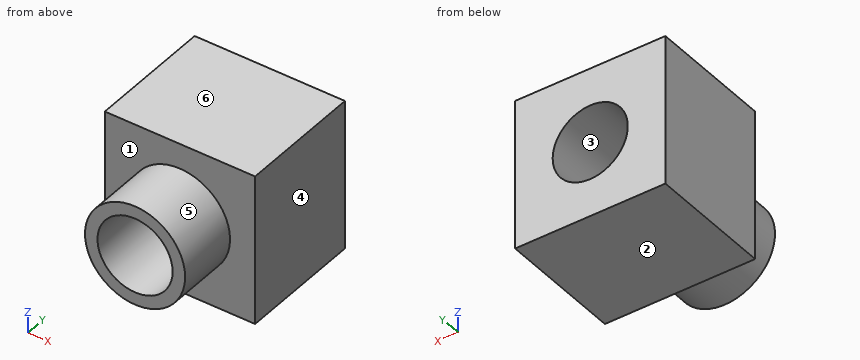
```python
from build123d import *

# Parameters (mm, degrees)
F0_W     = 600
F0_H     = 600
F1_DEPTH = 250
F2_R     = 200
F2_R_2   = 150
F3_DEPTH = 250
F4_R     = 150
F5_DEPTH = 1016


with BuildPart() as f1:
    # F0 (on Front) → F1 (new body, symmetric)
    with BuildSketch(Plane.XZ):
        Rectangle(F0_W, F0_H)
    extrude(amount=F1_DEPTH, both=True)

    # F2 (on face) → F3 (join)
    with BuildSketch(Plane.XZ.offset(250)):
        Circle(F2_R)
        Circle(F2_R_2, mode=Mode.SUBTRACT)
    extrude(amount=F3_DEPTH)

    # F4 (on face) → F5 (cut)
    with BuildSketch(Plane.XZ.offset(500)):
        Circle(F4_R)
    extrude(amount=-F5_DEPTH, mode=Mode.SUBTRACT)


solid = f1.part
```
Geometry check sheet. Reference: the model listing, model coordinates, mm. Face numbers are marked on the shaded views. A direction names the side the tool comes from. Coordinates: 2 decimals unless noted, no trailing zeros. Order: outer loops, then holes, each group sorted by start corner. A loop starts at its lowest first (then second) coordinate and runs counter-clockwise, first axis right, second up.
Item 1: Mould release check, pull along X, two halves, no side actions. Record for the marked faces 3, 4, 5 and 6: released by +X, released by -X, zero draft, split by the parting line, or undercut.
Item 2: Tool access check on the marked faces 1 and 2. Record the directions out of +Z, -Z, +X, -X, +Y, -Y that give a thin tool (end or side, any length) a straight path to the whole face; none if there is none.
Item 3: Section check D-D (z = 177). Enter the section's corners in (x, y), plus the area to 3 significant figures.
Item 4: Section check B-B (x = 0). Enter the section's corners in (y, z).
Item 5: Section check A-A (z = 0). Enter the section's corners in (x, y).
Item 6: Scan lines: line 1 along Z through (x, y) = (0, -46); line 2 along Z through (x, y) = (0, -340); line 3 along Y through (x, z) = (236.5, -69). Record each from-to range of solid material in increasing order.
Item 7: Section check C-C (y = -349). Enter the section's corners in (x, z).
Item 8: Depth check by flat-ended pin: pin 1 (3 mm diameter, centred on x = 96, y = -324, fed in from -Z); pin 2 (3 mm diameter, centred on y = -281, z = 30.5, fed in from -X). Enter the tip coordinate at first touch or a pass-through.
Check sheet entries:
1. face 3: undercut
1. face 4: released by +X
1. face 5: split by the parting line
1. face 6: zero draft
2. face 1: -Y
2. face 2: -Z, +X, -X, +Y, -Y
3. outline: (-300, -250) - (-93.12, -250) - (-93.12, -500) - (93.12, -500) - (93.12, -250) - (300, -250) - (300, 250) - (-300, 250) - close
3. area: 347,000 mm2
4. outline: (-500, -200) - (-250, -200) - (-250, -300) - (250, -300) - (250, -150) - (-500, -150) - close; (-500, 150) - (250, 150) - (250, 300) - (-250, 300) - (-250, 200) - (-500, 200) - close
5. outline: (-300, -250) - (-200, -250) - (-200, -500) - (-150, -500) - (-150, 250) - (-300, 250) - close; (150, -500) - (200, -500) - (200, -250) - (300, -250) - (300, 250) - (150, 250) - close
6. line 1: z = -300 to -150, 150 to 300
6. line 2: z = -200 to -150, 150 to 200
6. line 3: y = -250 to 250
7. outline: circle Ø400 at (0, 0); hole circle Ø300 at (0, 0)
8. pin 1: stops at z = -176.27
8. pin 2: stops at x = -197.89
